Can you work these out from the model? Positions are in its coordinate system, mm. A direction names the side the tool comes from. Coordinates: 2 decimals unless noted, no trailing zeros. Loops run counter-clockwise (first coordinate to the right, second up) from the corner with the lowest first, then second, coordinate; pieces in that order, holes last.
```python
from build123d import *

# Parameters (mm, degrees)
BOSS_EXTRUDE2_DEPTH   = 50
SHELL2_T              = -10
SKETCH2_R             = 12.5
CUT_EXTRUDE1_DEPTH    = 10
M5_TAPPED_HOLE1_D     = 4.2
M5_TAPPED_HOLE1_DEPTH = 10
M5_TAPPED_HOLE1_TIP   = 1.2618073
SKETCH7_R             = 2.5
BOSS_EXTRUDE3_DEPTH   = 20


with BuildPart() as part:
    # Sketch1 → Boss-Extrude2 (new body)
    with BuildSketch(Plane.XY):
        with BuildLine():
            Line((-71.001256012, 89.910155998), (375.818743988, 69.930121332))
            ThreePointArc((375.818743988, 69.930121332), (442.691743746, 0), (375.818743988, -69.930121332))
            Line((375.818743988, -69.930121332), (-71.001256012, -89.910155998))
            ThreePointArc((-71.001256012, -89.910155998), (-165.021684895, 0), (-71.001256012, 89.910155998))
        make_face()
    extrude(amount=BOSS_EXTRUDE2_DEPTH)

    # Shell2
    shell2_openings = [part.faces().sort_by_distance(p)[0] for p in [
        (145.621886707, 0, 50),
    ]]
    offset(amount=SHELL2_T, openings=shell2_openings, kind=Kind.INTERSECTION)

    # Sketch2 → Cut-Extrude1 (cut)
    with BuildSketch(Plane.XY.offset(10)):
        with Locations((-75.021684895, 0)):
            Circle(SKETCH2_R)
        with Locations((372.691743746, 0)):
            Circle(SKETCH2_R)
    extrude(amount=-CUT_EXTRUDE1_DEPTH, mode=Mode.SUBTRACT)

    # M5 Tapped Hole1
    with Locations(Plane.XY.offset(50)):
        with Locations((-160.021684895, 3.133929532), (-75.081342532, 85), (-75.021684895, -85), (437.691743746, 0), (372.686127316, -64.999999757), (372.691743746, 65), (151.962029668, 74.920138665), (151.962918886, -74.94005433)):
            Hole(M5_TAPPED_HOLE1_D / 2, depth=M5_TAPPED_HOLE1_DEPTH)
            with Locations((0, 0, -(M5_TAPPED_HOLE1_DEPTH + M5_TAPPED_HOLE1_TIP / 2))):  # 118° drill point
                Cone(0, M5_TAPPED_HOLE1_D / 2, M5_TAPPED_HOLE1_TIP, mode=Mode.SUBTRACT)

    # Sketch7 → Boss-Extrude3 (add)
    with BuildSketch(Plane(origin=(0, 0, 0), x_dir=(-1, 0, 0), z_dir=(0, 0, -1))):
        Polygon((-268.221462492, -5.800860149), (-109.826947867, -27.830102859), (-93.540881228, -30.095141618), (-90.785832397, -10.285807809), (-288.879170482, 17.264680503), (-291.634219314, -2.544653305), align=None)
        with Locations((-270.447361089, 4.604964768)):
            Circle(SKETCH7_R, mode=Mode.SUBTRACT)
        with Locations((-191.210025855, -6.415230557)):
            Circle(SKETCH7_R, mode=Mode.SUBTRACT)
        with Locations((-111.972690621, -17.435425882)):
            Circle(SKETCH7_R, mode=Mode.SUBTRACT)
    extrude(amount=BOSS_EXTRUDE3_DEPTH)


solid = part.part
```
(1) If I drill on probe 1 along Y at (x, z) = (203, -15.5); probe 2 along Z at (x, y) = (236.5, -50); probe 3 along Y at (x, z) = (26.5, 21), over which ranges is the centre line in solid material (lowest first)?
Check values:
probe 1: y = -14.87 to 5.32
probe 2: z = 0 to 10
probe 3: y = -85.55 to -75.54, 75.54 to 85.55
(2) I want a section at A-A on z = 20. Write out the boundary of the cut face in (x, y), then the cut area to 3 significant figures.
Check values:
outline: (-71, -89.91) - (375.82, -69.93) arc R70 ccw to (375.82, 69.93) - (-71, 89.91) arc R90 ccw (long way) to start; hole (-71.45, -79.92) - (375.37, -59.94) arc R60 ccw to (375.37, 59.94) - (-71.45, 79.92) arc R80 ccw (long way) to start
area: 13,700 mm2
(3) Which directions (+Z, -Z, +X, -X, +Y, -Y) give clear straight access to the entire face, cutting with the end or side of a thin tool? Please do faces 4 (the flat face through (148.83, 70.07, 29.72)), 5 (the flat face through (92.183, -20.329, -9.86)), 6 (the flat face through (188.446, 3.297, -9.86)).
Check values:
face 4: +Z
face 5: -Z, -X, -Y
face 6: -Z, -X, +Y
(4) I want a section at D-D on x = -113. Write out the boundary of the cut face in (y, z).
Check values:
outline: (-81.59, 0) - (81.59, 0) - (81.59, 50) - (70.41, 50) - (70.41, 10) - (-70.41, 10) - (-70.41, 50) - (-81.59, 50) - close
(5) If we mould it in two halves opening along X, with no side actions, what happens to faces 1 (the flat face through (163, 74, 50)), 2 (the flat face through (155.54, -79.78, 24.65)), 3 (the cylindrical face through (-87.51, 0.55, 5.07))? For each: released by +X, released by -X, zero draft, split by the parting line, or undercut.
Check values:
face 1: zero draft
face 2: released by +X
face 3: undercut
(6) I want a section at C-C on z = -7.5. Write out the boundary of the cut face in (x, y).
Check values:
outline: (90.79, -10.29) - (93.54, -30.1) - (291.63, -2.54) - (288.88, 17.26) - close; hole circle Ø5 at (111.97, -17.44); hole circle Ø5 at (191.21, -6.42); hole circle Ø5 at (270.45, 4.6)
(7) I'm going to push flat-ended pins straight in: pin 1 (5.5 mm diameter, centred on x = -160.02, y = 3.13, fed in from -Z); pin 2 (12 mm diameter, centred on x = 118.5, z = 21.5, fed in from +Y); pin 3 (4 mm diameter, centred on x = 437.69, y = 0, fed in from +Z). Where does each tip first touch, or does it pass through?
Check values:
pin 1: stops at z = 0
pin 2: stops at y = 81.7
pin 3: stops at z = 39.94
(8) I want a section at B-B on x = 2. Write out the boundary of the cut face in (y, z).
Check values:
outline: (-86.65, 0) - (86.65, 0) - (86.65, 50) - (76.64, 50) - (76.64, 10) - (-76.64, 10) - (-76.64, 50) - (-86.65, 50) - close
